Here's how the part is built. I have some questions about the finished solid (model axes, mm). A direction names the side the tool comes from. Give positions to 0.01 mm unless a question says otherwise; leave off trailing zeros. Loops run counter-clockwise (first coordinate to the right, second up) from the corner with the lowest first, then second, coordinate; pieces in that order, holes last. Notation, with made-up numbers: (16.5, -13.5) - (68.5, -13.5) arc R24 cw to (68.5, 6.5) - close; hole circle Ø3 at (-35.75, -31). An arc over 180 degrees is marked (long way). Use a Markdown table: item, result.
from build123d import *

# Parameters (mm, degrees)
SKETCH1_W           = 181.102
SKETCH1_H           = 76.454
BOSS_EXTRUDE1_DEPTH = 166.878
SKETCH2_W           = 38.1
SKETCH2_H           = 19.05
CUT_EXTRUDE1_DEPTH  = 12.7
SKETCH3_R           = 3.175
BOSS_EXTRUDE2_DEPTH = 6.35


with BuildPart() as part:
    # Sketch1 → Boss-Extrude1 (new body)
    with BuildSketch(Plane(origin=(0, 0, 0), x_dir=(1, 0, 0), z_dir=(0, 1, 0))):
        with Locations((-20.72278737, -46.488845277)):
            Rectangle(SKETCH1_W, SKETCH1_H)
    extrude(amount=BOSS_EXTRUDE1_DEPTH)

    # Sketch2 → Cut-Extrude1 (cut)
    with BuildSketch(Plane(origin=(0, 166.878, 0), x_dir=(1, 0, 0), z_dir=(0, 1, 0))):
        with Locations((-92.22378737, -75.190845277)):
            Rectangle(SKETCH2_W, SKETCH2_H)
        with Locations((50.77821263, -75.190845277)):
            Rectangle(SKETCH2_W, SKETCH2_H)
    extrude(amount=-CUT_EXTRUDE1_DEPTH, mode=Mode.SUBTRACT)

    # Sketch3 → Boss-Extrude2 (add)
    with BuildSketch(Plane(origin=(0, 154.178, 0), x_dir=(1, 0, 0), z_dir=(0, 1, 0))):
        with Locations((63.47821263, -75.443767272)):
            Circle(SKETCH3_R)
        with Locations((-104.92378737, -75.443767272)):
            Circle(SKETCH3_R)
    extrude(amount=BOSS_EXTRUDE2_DEPTH)


solid = part.part
(1) Will these pins go through, and if not, where does the flat tip stop? pin 1 (14 mm diameter, centred on y = 162.5, z = 80, fed in from +X); pin 2 (14 mm diameter, centred on x = 55, y = 162, fed in from +Z); pin 3 (4 mm diameter, centred on x = -86, y = 158.5, fed in from +Z); pin 4 (5 mm diameter, centred on x = -61.5, z = 23.5, fed in from -Y).
A:
| item | result |
|---|---|
| pin 1 | x = 66.65 |
| pin 2 | z = 78.17 |
| pin 3 | z = 65.67 |
| pin 4 | y = 0 |
(2) We'd pull the mould along X, two halves only. Please class faces 1 (the face through (69.828, 82, 47)), 2 (the face through (63, 160.528, 75)), 3 (the face through (31.728, 161, 75)): pulls with the +X half, pulls with the -X half, needs draft (parallel to the pull), parting line crosses it, or undercut.
A:
| item | result |
|---|---|
| face 1 | pulls with the +X half |
| face 2 | needs draft |
| face 3 | undercut |
(3) Suppose I cut it at A-A on x = 45. Write out the boundary of the cut face in (y, z), plus the area to 3 significant figures.
A:
| item | result |
|---|---|
| outline | (0, 8.26) - (166.88, 8.26) - (166.88, 65.67) - (154.18, 65.67) - (154.18, 84.72) - (0, 84.72) - close |
| area | 12,500 mm2 |
(4) On a 3-axis mill with a long thin cutter (end or side, diameter ignored), from which of +Z, -Z, +X, -X, +Y, -Y can I reach the whole of each face in a straight line? I mean faces 4 (the face through (61.138, 157.309, 73.298)), 5 (the face through (-22, 0, 46)), 6 (the face through (-73.174, 161, 75)), 7 (the face through (-22, 82, 8.262)), 8 (the face through (-105, 160.528, 75)). Say none if no direction works.
A:
| item | result |
|---|---|
| face 4 | +Y |
| face 5 | +Z, -Z, +X, -X, -Y |
| face 6 | +Z, +Y |
| face 7 | -Z, +X, -X, +Y, -Y |
| face 8 | +Z, -X, +Y |
(5) If I drill on line 1 (Y direction, x = 42.5, z = 78); line 2 (X direction, y = 156.5, z = 67), over which ranges is the centre line in solid material (lowest first)?
A:
| item | result |
|---|---|
| line 1 | 0 to 154.18 |
| line 2 | -73.17 to 31.73 |
